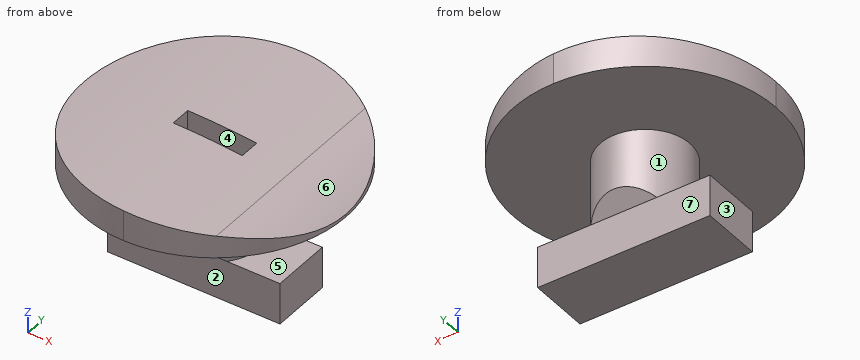
Autodesk Inventor part; units mm, degrees
ref_plane "YZ Plane" through (0, 0, 0) normal (1, 0, 0) x (0, 1, 0)
ref_plane "XZ Plane" through (0, 0, 0) normal (0, 1, 0) x (-1, 0, 0)
ref_plane "XY Plane" through (0, 0, 0) normal (0, 0, 1) x (1, 0, 0)
sketch "Sketch1" plane through (0, 0, 0) normal (0, 0, 1) x (1, 0, 0)
  circle A0 centre (0, 0) radius 9.5
  line L0 (-2.5, 0.75) -> (2.5, 0.75)
  line L1 (2.5, 0.75) -> (2.5, -0.75)
  line L2 (2.5, -0.75) -> (-2.5, -0.75)
  line L3 (-2.5, -0.75) -> (-2.5, 0.75)
  line L4 (0, -0.75) -> (0, 0.75) construction
  line L5 (0, -13.3) -> (0, 13.3) construction
  line L6 (-13.3, 0) -> (13.3, 0) construction
  point P0 (2.5, 0)
  dimension "d0" = 19
  dimension "d1" = 1.5
  dimension "d2" = 5
extrude "Extrusion1" add sketch "Sketch1" along normal blind 2.3
sketch "Sketch2" plane through (0, 0, 0) normal (0, 1, 0) x (-1, 0, 0)
  line L0 (-2.5, 2.3) -> (2.5, 2.3) construction
  line L1 (2.5, 2.3) -> (-2.5, 2.3) construction
  line L2 (-9.5, 2.3) -> (9.5, 2.3) construction
  line L3 (-9.5, 2.3) -> (9.5, 2.3) construction
  line L4 (-2.5, 0) -> (2.5, 0) construction
  line L5 (2.5, 0) -> (-2.5, 0) construction
  line L6 (-9.5, 0) -> (9.5, 0) construction
  line L7 (-9.5, 0) -> (-9.5, 0.2)
  line L8 (-9.5, 0) -> (9.5, 0)
  line L9 (9.5, 0) -> (9.5, 1.9)
  arc A0 (-5.5, 1.6114) -> (-9.5, 0.2) centre (-3.57, -10.2324) ccw
  arc A1 (17.6587, 0.2303) -> (-5.5, 1.6114) centre (3.0073, -50.5943) ccw
  point P0 (0, 0)
  dimension "d5" = 12
  dimension "d6" = 0.2
  dimension "d8" = 1.9
  dimension "d9" = 4
extrude "Extrusion2" cut sketch "Sketch2" along normal through all both and the other way through all keep common part
sketch "Sketch3" plane through (0, 0, 0) normal (0, 1, 0) x (-1, 0, 0)
  line L0 (-2.5, 0) -> (2.5, 0) construction
  line L1 (2.5, 0) -> (-2.5, 0) construction
  line L2 (-9.5, 0) -> (9.5, 0) construction
  line L3 (-3.25, 0) -> (0, 0)
  line L4 (0, 0) -> (0, -5)
  line L5 (0, -5) -> (-3.25, -5)
  line L6 (-3.25, -5) -> (-3.25, 0)
  point P0 (0, 0)
  dimension "d12" = 3.25
  dimension "d13" = 5
revolve "Revolution1" add sketch "Sketch3" angle 360 about axis through (0, 0, 0) along (0, 0, -1)
sketch "Sketch4" plane through (0, 0, 0) normal (0, 1, 0) x (-1, 0, 0)
  line L0 (-6.25, -5) -> (6.25, -5)
  line L1 (6.25, -5) -> (6.25, -8)
  line L2 (6.25, -8) -> (-6.25, -8)
  line L3 (-6.25, -8) -> (-6.25, -5)
  line L4 (0, -12.0667) -> (0, 4.6989) construction
  line L5 (3.25, -5) -> (-3.25, -5) construction
  point P0 (0, 0)
  point P1 (0, -5)
  dimension "d16" = 3
  dimension "d17" = 12.5
extrude "Extrusion3" add sketch "Sketch4" along normal blind 2.2 and the other way blind 2.2
sketch "Sketch5" plane through (0, 0, 0) normal (1, 0, 0) x (0, 1, 0)
  line L0 (2.2, -5) -> (2.2, -8) construction
  line L1 (2.2, -8) -> (2.2, -5) construction
  line L2 (3.25, -5) -> (3.25, 0) construction
  line L3 (-3.25, -5) -> (-3.25, 0) construction
  line L4 (-2.2, -5) -> (-2.2, -8) construction
  line L5 (-2.2, -8) -> (-2.2, -5) construction
  line L6 (-2.2, -5) -> (-3.25, -4)
  line L7 (2.2, -5) -> (3.25, -4)
  line L8 (3.25, -4) -> (-3.25, -4)
  line L9 (-2.2, -5) -> (-3.25, -5)
  line L10 (-3.25, -5) -> (-3.25, -4)
  line L11 (2.2, -5) -> (3.25, -5)
  line L12 (3.25, -4) -> (3.25, -5)
  point P0 (0, 0)
  point P1 (2.2, -5)
  point P2 (2.2, -5)
  dimension "d23" = 1
extrude "Extrusion4" cut sketch "Sketch5" along normal through all both and the other way through all
properties part number "CRX brake light housing retainer"
Could you check a few things on this model? Use its own coordinates, in mm. Face numbers are marked on the shaded views. A direction names the side the tool comes from. Give positions to 0.01 mm unless a question says otherwise; leave off trailing zeros. Loops run counter-clockwise (first coordinate to the right, second up) from the corner with the lowest first, then second, coordinate; pieces in that order, holes last. Notation, with made-up numbers: (-22, 28) -> (33, 28) arc R18 cw to (33, 54) -> close; hole circle Ø8 at (-19.75, 36.5). An arc over 180 degrees is marked (long way). Answer as CSV lines item,"result". Start each with the question number.
(1) I'm going to push flat-ended pins straight in: pin 1 Ø1.2 at (x, y) = (1, 0.5) entering from +Z; pin 2 Ø2 at (x, z) = (-4.5, -3) entering from +Y; pin 3 Ø1.5 at (y, z) = (0, -6.5) entering from +X; pin 4 Ø1.5 at (x, z) = (1, -7) entering from +Y. Where does each tip first touch, or does it pass through?
(2) Which directions (+Z, -Z, +X, -X, +Y, -Y) give clear straight access to the entire face, cutting with the end or side of a thin tool? Please do the marked faces 1, 2, 3 and 4.
(3) If we section it at C-C on z = -3: Write out the boundary of the cut face in (x, y).
(4) We'd pull the mould along Z, two halves only. Please class the marked faces 5, 6 and 7: released by +Z, released by -Z, zero draft, split by the parting line, or undercut.
(5) I need wall thicknesses on probe 1 along Z at (x, y) = (5.5, 6.5); probe 2 along X at (y, z) = (1.25, -6.75); probe 3 along Y at (x, z) = (-5.5, -6). Which ranges of each line are inside material? Lowest first, please.
(6) If we section it at B-B on y = -1.25: Write out the boundary of the cut face in (x, z).
(7) If we section it at A-A on x = 4.25: Write out the boundary of the cut face in (y, z).
(8) If we section it at D-D on x = -1.25: Write out the boundary of the cut face in (y, z), then the cut area to 3 significant figures.
Computed:
1,pin 1,"stops at z = 2.19"
1,pin 2,"passes through"
1,pin 3,"stops at x = 6.25"
1,pin 4,"stops at y = 2.2"
2,face 1,"none"
2,face 2,"-Z, +X, -X, -Y"
2,face 3,"-Z, -X, +Y, -Y"
2,face 4,"+Z"
3,outline,"circle Ø6.5 at (0, 0)"
4,face 5,"undercut"
4,face 6,"released by +Z"
4,face 7,"zero draft"
5,probe 1,"z = 0 to 1.61"
5,probe 2,"x = -6.25 to 6.25"
5,probe 3,"y = -2.2 to 2.2"
6,outline,"(-9.42, 0) -> (-3, 0) -> (-3, -5) -> (-6.25, -5) -> (-6.25, -8) -> (6.25, -8) -> (6.25, -5) -> (3, -5) -> (3, 0) -> (9.42, 0) -> (9.42, 0.25) arc R12 ccw to (5.5, 1.61) arc R52.9 ccw to (-9.42, 1.91) -> close"
7,outline,"(-8.5, 0) -> (8.5, 0) -> (8.5, 1.8) -> (-8.5, 1.8) -> close; (-2.2, -8) -> (2.2, -8) -> (2.2, -5) -> (-2.2, -5) -> close"
8,outline,"(-9.42, 0) -> (-3, 0) -> (-3, -4.24) -> (-2.2, -5) -> (-2.2, -8) -> (2.2, -8) -> (2.2, -5) -> (3, -4.24) -> (3, 0) -> (9.42, 0) -> (9.42, 2.27) -> (0.75, 2.27) -> (0.75, 0) -> (-0.75, 0) -> (-0.75, 2.27) -> (-9.42, 2.27) -> close"
8,area,"82.0 mm2"
